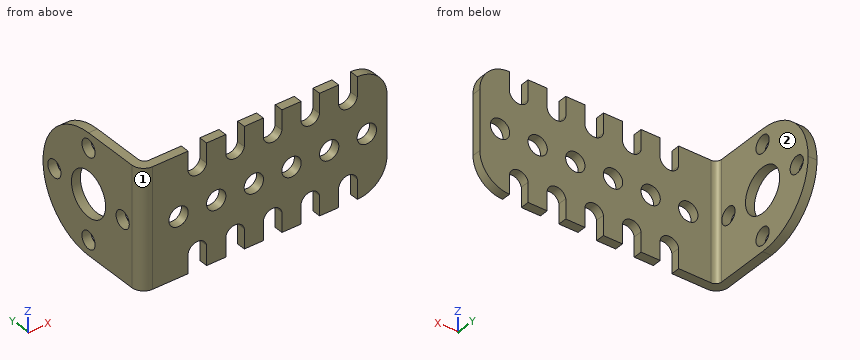
from build123d import *

# Parameters (mm, degrees)
BOSS_EXTRUDE1_DEPTH   = 20
FILLET1_R             = 2
FILLET2_R             = 1
CUT_EXTRUDE1_DEPTH    = 51.222007128
F_4_CLEARANCE_HOLE1_D = 3.2639
FILLET3_R             = 5
FILLET4_R             = 10
SKETCH7_R             = 3.75
SKETCH7_R_2           = 1.45
CUT_EXTRUDE2_DEPTH    = 51.83797793


with BuildPart() as part:
    # Sketch1 → Boss-Extrude1 (new body)
    with BuildSketch(Plane.XY):
        Polygon((0, 0), (41.5, 0), (41.5, 1.5), (1.5, 1.5), (1.5, 21.5), (0, 21.5), align=None)
    extrude(amount=BOSS_EXTRUDE1_DEPTH)

    # Fillet1
    fillet1_edges = [part.edges().sort_by_distance(p)[0] for p in [
        (0, 0, 10),
    ]]
    fillet(fillet1_edges, radius=FILLET1_R)

    # Fillet2
    fillet2_edges = [part.edges().sort_by_distance(p)[0] for p in [
        (1.5, 1.5, 10),
    ]]
    fillet(fillet2_edges, radius=FILLET2_R)

    # Sketch3 → Cut-Extrude1 (cut, through all)
    with BuildSketch(Plane(origin=(0, 1.5, 0), x_dir=(1, 0, 0), z_dir=(0, 1, 0))):
        with BuildLine():
            Line((7.96, 0), (11.09, 0))
            Line((11.09, 0), (11.09, -3.307162367))
            ThreePointArc((11.09, -3.307162367), (9.525, -4.594858526), (7.96, -3.307162367))
            Line((7.96, -3.307162367), (7.96, 0))
        make_face()
        with BuildLine():
            Line((14.31, 0), (17.44, 0))
            Line((17.44, 0), (17.44, -3.307162367))
            ThreePointArc((17.44, -3.307162367), (15.875, -4.594858526), (14.31, -3.307162367))
            Line((14.31, -3.307162367), (14.31, 0))
        make_face()
        with BuildLine():
            Line((20.66, 0), (23.79, 0))
            Line((23.79, 0), (23.79, -3.307162367))
            ThreePointArc((23.79, -3.307162367), (22.225, -4.594858526), (20.66, -3.307162367))
            Line((20.66, -3.307162367), (20.66, 0))
        make_face()
        with BuildLine():
            Line((27.01, 0), (30.14, 0))
            Line((30.14, 0), (30.14, -3.307162367))
            ThreePointArc((30.14, -3.307162367), (28.575, -4.594858526), (27.01, -3.307162367))
            Line((27.01, -3.307162367), (27.01, 0))
        make_face()
        with BuildLine():
            Line((33.36, 0), (36.49, 0))
            Line((36.49, 0), (36.49, -3.307162367))
            ThreePointArc((36.49, -3.307162367), (34.925, -4.594858526), (33.36, -3.307162367))
            Line((33.36, -3.307162367), (33.36, 0))
        make_face()
        with BuildLine():
            Line((36.49, -20), (36.49, -16.692837633))
            ThreePointArc((36.49, -16.692837633), (34.925, -15.405141474), (33.36, -16.692837633))
            Line((33.36, -16.692837633), (33.36, -20))
            Line((33.36, -20), (36.49, -20))
        make_face()
        with BuildLine():
            Line((30.14, -20), (30.14, -16.692837633))
            ThreePointArc((30.14, -16.692837633), (28.575, -15.405141474), (27.01, -16.692837633))
            Line((27.01, -16.692837633), (27.01, -20))
            Line((27.01, -20), (30.14, -20))
        make_face()
        with BuildLine():
            Line((23.79, -20), (23.79, -16.692837633))
            ThreePointArc((23.79, -16.692837633), (22.225, -15.405141474), (20.66, -16.692837633))
            Line((20.66, -16.692837633), (20.66, -20))
            Line((20.66, -20), (23.79, -20))
        make_face()
        with BuildLine():
            Line((17.44, -20), (17.44, -16.692837633))
            ThreePointArc((17.44, -16.692837633), (15.875, -15.405141474), (14.31, -16.692837633))
            Line((14.31, -16.692837633), (14.31, -20))
            Line((14.31, -20), (17.44, -20))
        make_face()
        with BuildLine():
            Line((11.09, -20), (11.09, -16.692837633))
            ThreePointArc((11.09, -16.692837633), (9.525, -15.405141474), (7.96, -16.692837633))
            Line((7.96, -16.692837633), (7.96, -20))
            Line((7.96, -20), (11.09, -20))
        make_face()
    extrude(amount=-CUT_EXTRUDE1_DEPTH, mode=Mode.SUBTRACT)

    # #4 Clearance Hole1 (through all)
    with Locations(Plane(origin=(0, 1.5, 0), x_dir=(1, 0, 0), z_dir=(0, 1, 0))):
        with Locations((6.35, -10), (12.7, -10), (25.4, -10), (31.75, -10), (38.1, -10), (19.05, -10)):
            Hole(F_4_CLEARANCE_HOLE1_D / 2)

    # Fillet3
    fillet3_edges = [part.edges().sort_by_distance(p)[0] for p in [
        (41.5, 0.75, 20),
        (41.5, 0.75, 0),
    ]]
    fillet(fillet3_edges, radius=FILLET3_R)

    # Fillet4
    fillet4_edges = [part.edges().sort_by_distance(p)[0] for p in [
        (0.75, 21.5, 0),
        (0.75, 21.5, 20),
    ]]
    fillet(fillet4_edges, radius=FILLET4_R - 0.0001)  # a hair under: the kernel refuses the full size

    # Sketch7 → Cut-Extrude2 (cut, through all)
    with BuildSketch(Plane.ZY):
        with Locations(Location((10, 11.5, 0), (0, 0, 270))):
            Circle(SKETCH7_R)
        with Locations(Location((10, 19, 0), (0, 0, 270))):
            Circle(SKETCH7_R_2)
        with Locations(Location((17.5, 11.5, 0), (0, 0, 270))):
            Circle(SKETCH7_R_2)
        with Locations(Location((10, 4, 0), (0, 0, 270))):
            Circle(SKETCH7_R_2)
        with Locations(Location((2.5, 11.5, 0), (0, 0, 270))):
            Circle(SKETCH7_R_2)
    extrude(amount=-CUT_EXTRUDE2_DEPTH, mode=Mode.SUBTRACT)


solid = part.part
Could you check a few things on this model? Use its own coordinates, in mm. Face numbers are marked on the shaded views. A direction names the side the tool comes from. Round coordinates to 2 decimals unless told otherwise and drop trailing zeros. Write each loop counter-clockwise with the first axis right and the second up, starting at its lowest first coordinate (ties: lowest second). Pieces come first, ordered by that corner, then holes. Notation, with made-up numbers: (-23, 62) - (16, 62) arc R21 ccw to (16, 69) - close; hole circle Ø1 at (3, 4.5). An arc over 180 degrees is marked (long way). Put each result on its own line as item: value. Start each with the question number.
(1) I want a section at D-D, the plane z = 7. Please give me the cut outline in (x, y).
(2) I want a section at A-A, the plane y = 4. Please give me the cut outline in (x, z).
(3) I want a section at C-C, the plane z = 18. Give the number of separate pieces and of enclosed holes in the cut face, plus the area to 3 significant figures.
(4) I need wall thicknesses on probe 1 along Z at (x, y) = (0.75, 11.5); probe 2 along Z at (x, y) = (12.7, 1.2); probe 3 along Z at (x, y) = (1.2, 4). Which ranges of each line are inside material? Lowest first, please.
(5) Will these pins go through, and if not, where does the flat tip stop? pin 1 (3 mm diameter, centred on x = 10.5, z = 12.5, fed in from +Y); pin 2 (2 mm diameter, centred on x = 38.1, z = 10, fed in from +Y); pin 3 (1.2 mm diameter, centred on y = 1, z = 1, fed in from +X); pin 4 (1.2 mm diameter, centred on y = 0.5, z = 1, fed in from -X).
(6) For the marked faces 1 and 2, which set-ups out of +Z, -Z, +X, -X, +Y, -Y let a thin tool reach every point of the face, with its end or its side?
(7) I want a section at B-B, the plane x = 25.4. Please give me the cut outline in (y, z).
Here are the results:
1. outline: (0, 2) arc R2 ccw to (2, 0) - (41.5, 0) - (41.5, 1.5) - (2.5, 1.5) arc R1 cw to (1.5, 2.5) - (1.5, 9.25) - (0, 9.25) - close; (0, 13.75) - (1.5, 13.75) - (1.5, 21.04) - (0, 21.04) - close
2. outline: (0, 0) - (1.5, 0) - (1.5, 8.55) - (0, 8.55) - close; (0, 11.45) - (1.5, 11.45) - (1.5, 20) - (0, 20) - close
3. separate pieces: 7
3. enclosed holes: 0
3. area: 56.5 mm^2
4. probe 1: z = 0 to 1.05, 3.95 to 6.25, 13.75 to 16.05, 18.95 to 20
4. probe 2: z = 0 to 8.37, 11.63 to 20
4. probe 3: z = 0 to 8.55, 11.45 to 20
5. pin 1: stops at y = 1.5
5. pin 2: passes through
5. pin 3: stops at x = 40.17
5. pin 4: stops at x = 0.21
6. face 1: +Z, -Z, -X, -Y
6. face 2: +Z, -Z, +X, +Y
7. outline: (0, 0) - (1.5, 0) - (1.5, 8.37) - (0, 8.37) - close; (0, 11.63) - (1.5, 11.63) - (1.5, 20) - (0, 20) - close
